Here's how the part is built. I have some questions about the finished solid (model axes, mm). Face numbers are marked on the shaded views. A direction names the side the tool comes from. Coordinates: 2 decimals unless noted, no trailing zeros. Loops run counter-clockwise (first coordinate to the right, second up) from the corner with the lowest first, then second, coordinate; pieces in that order, holes last. Notation, with made-up numbers: M 69.5,46.25 L 122.5,46.25 A17 ccw 122.5,51.25 Z; hole C 5.5,53 d8. An arc over 180 degrees is marked long. Use CSV: the item, a comma, the result in double quotes. Start each with the question number.
Q1. Please list where these lines run through material, in increasing order: probe 1 along X at (y, z) = (-114, 72); probe 2 along Y at (x, z) = (88.9, 76.5); probe 3 along Z at (x, y) = (29, 36). Write a range as [from, to].
Q2. If we section it at B-B (y = 11.5): Please give me the cut outline in (x, z), and give its area (3 significant figures).
Q3. Which directions (+Z, -Z, +X, -X, +Y, -Y) give clear straight access to the entire face, cutting with the end or side of a thin tool? Please do the marked faces 1, 2, 3 and 4.
Q4. If we mould it in two halves opening along Y, with no side actions, what happens to the marked faces 5, 6 and 7? For each: +Y half, -Y half, draft (parallel to the pull), parting line (faces both ways), or undercut.
Q5. If we section it at D-D (x = -84.5): Please give me the cut outline in (y, z).
Q6. For pin 1 Ø6 at (x, y) = (48, -30.5) entering from -Z; pin 2 Ø3 at (y, z) = (26.5, -16) entering from -X; pin 3 Ø4 at (x, z) = (-8.5, -15) entering from -Y, each with a flat end and sliding along its axis, tell me the tip position at first contact or that it passes through.
Q7. If we section it at A-A (x = 0): Please give me the cut outline in (y, z), and give its area (3 significant figures).
Q8. If we section it at C-C (y = -114.3): Please give me the cut outline in (x, z).
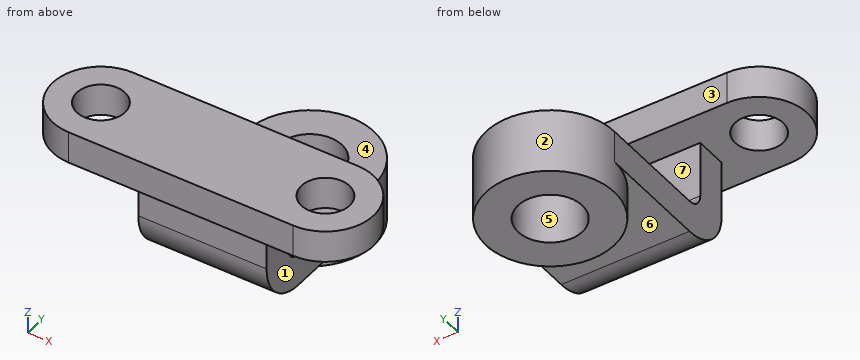
Autodesk Inventor part; units mm, degrees
ref_plane "YZ Plane" through (0, 0, 0) normal (1, 0, 0) x (0, 1, 0)
ref_plane "XZ Plane" through (0, 0, 0) normal (0, 1, 0) x (-1, 0, 0)
ref_plane "XY Plane" through (0, 0, 0) normal (0, 0, 1) x (1, 0, 0)
sketch "Sketch1" plane through (0, 0, 0) normal (0, 0, 1) x (1, 0, 0)
  circle A0 centre (0, 0) radius 25.4
  circle A1 centre (0, 0) radius 50.8
  dimension "d0" = 50.8
  dimension "d1" = 101.6
extrude "Extrusion1" add sketch "Sketch1" against normal blind 50.8
sketch "Sketch2" plane through (0, 0, 0) normal (0, 0, 1) x (1, 0, 0)
  circle A0 centre (0, 0) radius 50.8
  line L0 (50.8, 0) -> (50.8, -127)
  line L1 (-50.8, 0) -> (-50.8, -127)
  line L2 (-50.8, -127) -> (50.8, -127)
  circle A1 centre (0, 0) radius 50.8
  dimension "d4" = 127
  dimension "d5" = 127
  dimension "d6" = 101.6
extrude "Extrusion2" add sketch "Sketch2" against normal blind 25.4 contours L0 L2 L1 A0
sketch "Sketch3" plane through (50.8, -127, 0) normal (1, 0, 0) x (0, 0, -1)
  line L0 (0, 0) -> (-57.15, 0)
  line L1 (-57.15, 0) -> (-57.15, 25.4)
  line L2 (-57.15, 25.4) -> (0, 25.4)
  line L3 (0, 25.4) -> (0, 0)
  point P0 (0, 127)
  dimension "d9" = 57.15
  dimension "d10" = 25.4
extrude "Extrusion3" add sketch "Sketch3" against normal blind 101.6
fillet "Fillet1" radius 12.7 1 edges at (0, -101.6, 0)
fillet "Fillet2" radius 38.1 1 edges at (0, -127, -25.4)
sketch "Sketch4" plane through (50.8, -127, 57.15) normal (0, 0, 1) x (1, 0, 0)
  line L0 (-139.7001, 50.8) -> (38.0999, 50.8)
  line L1 (-139.7001, -25.4) -> (38.1001, -25.4)
  arc A0 (-139.7001, 50.8) -> (-139.7001, -25.4) centre (-139.7001, 12.7) ccw
  arc A1 (38.1001, -25.4) -> (38.0999, 50.8) centre (38.1, 12.7) ccw
  line L2 (0, 0) -> (-101.6, 0)
  line L3 (-50.8, 0) -> (-50.8, -12.1544)
  line L4 (-50.8, -25.4) -> (-50.8, -31.0464)
  circle A2 centre (-139.7001, 12.7) radius 19.05
  circle A3 centre (38.1, 12.7) radius 19.05
  point P0 (-50.8, 127)
  dimension "d15" = 177.8
  dimension "d16" = 76.2
  dimension "d17" = 38.1
  dimension "d18" = 38.1
  dimension "d20" = 25.4
  dimension "d21" = 0
  dimension "d22" = 38.1
  dimension "d23" = 38.1
extrude "Extrusion4" add sketch "Sketch4" along normal blind 25.4
equation "\"d1\" = 2 * d0"
equation "\"d5\" = d4"
equation "\"d17\" = 0.5 * d16"
equation "\"d18\" = d17"
equation "\"d23\" = d22"
properties part number "HW 5 Part 6"
Results below:
1,probe 1,"[-127, -107.95], [-69.85, 69.85], [107.95, 127]"
1,probe 2,"[-152.4, -133.35], [-95.25, -76.2]"
1,probe 3,"[-50.8, 0]"
2,outline,"M -49.48,-50.8 L -22.65,-50.8 L -22.65,0 L -49.48,0 Z; M 22.65,-50.8 L 49.48,-50.8 L 49.48,0 L 22.65,0 Z"
2,area,"2,730 mm^2"
3,face 1,"-Z, +X, +Y, -Y"
3,face 2,"-Z"
3,face 3,"+Z, +X, -X, +Y"
3,face 4,"+X, -X, +Y"
4,face 5,"undercut"
4,face 6,"draft"
4,face 7,"+Y half"
5,outline,"M -152.4,57.15 L -132.83,57.15 L -132.83,82.55 L -152.4,82.55 Z; M -95.77,57.15 L -76.2,57.15 L -76.2,82.55 L -95.77,82.55 Z"
6,pin 1,"z = -25.4"
6,pin 2,"x = -44.22"
6,pin 3,"y = -117.03"
7,outline,"M -152.4,57.15 L -127,57.15 L -127,12.7 A38.1 ccw -88.9,-25.4 L -50.8,-25.4 L -50.8,-50.8 L -25.4,-50.8 L -25.4,0 L -88.9,0 A12.7 cw -101.6,12.7 L -101.6,57.15 L -76.2,57.15 L -76.2,82.55 L -152.4,82.55 Z; M 25.4,-50.8 L 50.8,-50.8 L 50.8,0 L 25.4,0 Z"
7,area,"7,630 mm^2"
8,outline,"M -127,57.15 L -107.95,57.15 L -107.95,82.55 L -127,82.55 Z; M -69.85,57.15 L -50.8,57.15 L -50.8,-15.7 L 50.8,-15.7 L 50.8,57.15 L 69.85,57.15 L 69.85,82.55 L -69.85,82.55 Z; M 107.95,57.15 L 127,57.15 L 127,82.55 L 107.95,82.55 Z"
